Source: CAD feature listing. Evaluate the final solid. Frame: model axes, mm. A direction names the side the tool comes from. Give positions to 0.01 mm unless a question says otherwise; leave off trailing zeros. Write each loop counter-clockwise with the first axis right and the second up, starting at its lowest first coordinate (ties: lowest second). Pieces come first, ordered by that corner, then holes. Notation, with made-up numbers: (89, 47) -> (112, 47) arc R22 ccw to (112, 59) -> close; hole circle Ø7 at (58, -38). An arc over 180 degrees is marked (long way). Use one line per item in the form item = value. Start each with the question number.
(1) Cut plane B-B, the plane x = 0. Output: boundary loops of the cut face in (y, z) (3 decimals), and give its area (3 significant figures).
(2) Set-up query: faces 4 (the face through (24, 4, -15)), 5 (the face through (20.724, 3.218, -20.751)), 6 (the face through (-21, 5.5, -21)). Return all of +Z, -Z, +X, -X, +Y, -Y with unobstructed straight access to the full face (end or side cutting, diameter ignored); none if empty.
(3) Cut plane C-C, the plane x = -5. Output: boundary loops of the cut face in (y, z), and give its area (3 significant figures).
(4) Cut plane A-A, the plane y = 12. Output: boundary loops of the cut face in (x, z), and give its area (3 significant figures).
(5) Material intervals for line 1 along X through (y, z) = (14, -0.5); line 2 along Z through (x, y) = (-14, 14.5), sorted ascending. Write a range as from..to.
(6) Cut plane D-D, the plane x = 15.5. Output: boundary loops of the cut face in (y, z), and give its area (3 significant figures).
(7) Draft query along X for faces 1 (the face through (24.5, 11, 0)), 2 (the face through (-0.958, 0.493, -21.084)), 3 (the face through (24, 4, 15)). Return one class per face: pulls with the +X half, pulls with the -X half, needs draft (parallel to the pull), parting line crosses it, or undercut.
(8) First-contact query: P1, Ø0.6, axis at x = -23.5, y = 11, coming from the +Z side; P2, Ø1.5, axis at x = -17, z = -4, coming from the +Y side; P3, Ø1.5, axis at x = 13.5, z = -19.5, coming from the -Y side; P4, Ø0.5, axis at y = 4, z = -22.5, coming from the +X side. Flat tips, straight axial feed; report the tip coordinate or a pass-through.
from build123d import *

# Parameters (mm, degrees)
EXTRUDE_1_DEPTH                = 19
SKETCH_1_3_R                   = 1.75
EXTRUDE_1_2_DEPTH              = 1
HOLE_WIZARD_M2_5_1_D           = 3.1
HOLE_WIZARD_M2_5_1_DEPTH       = 10
HOLE_WIZARD_M2_5_1_CSINK_D     = 5.5
HOLE_WIZARD_M2_5_1_CSINK_ANGLE = 90
HOLE_WIZARD_M2_5_1_TIP         = 0.931333959
SKETCH_4_R                     = 2.5
SKETCH_4_R_2                   = 1.75
SKETCH_4_W                     = 27
SKETCH_4_H                     = 26.512923835
CUT_EXTRUDE_1_DEPTH            = 143
CUT_EXTRUDE_2_DEPTH            = 21
CUT_EXTRUDE_4_DEPTH            = 27
EXTRUDE_2_DEPTH                = 4.5
CUT_EXTRUDE_START              = -0.8
SKETCH_9_W                     = 7.872983346
SKETCH_9_H                     = 13
SKETCH_9_W_2                   = 6.872983346
CUT_EXTRUDE_5_DEPTH            = 0.8


with BuildPart() as part:
    # 草图1 → Extrude 1 (new body)
    with BuildSketch(Plane(origin=(0, 0, 0), x_dir=(1, 0, 0), z_dir=(0, 1, 0))):
        with BuildLine():
            Line((-24.5, 21.2), (-24.5, -21.2))
            ThreePointArc((-24.5, -21.2), (-23.533452378, -23.533452378), (-21.2, -24.5))
            Line((-21.2, -24.5), (21.2, -24.5))
            ThreePointArc((21.2, -24.5), (23.533452378, -23.533452378), (24.5, -21.2))
            Line((24.5, -21.2), (24.5, 21.2))
            ThreePointArc((24.5, 21.2), (23.533452378, 23.533452378), (21.2, 24.5))
            Line((21.2, 24.5), (-21.2, 24.5))
            ThreePointArc((-21.2, 24.5), (-23.533452378, 23.533452378), (-24.5, 21.2))
        make_face()
        with BuildLine():
            Line((-23, 21.2), (-23, -21.2))
            ThreePointArc((-23, -21.2), (-22.472792206, -22.472792206), (-21.2, -23))
            Line((-21.2, -23), (21.2, -23))
            ThreePointArc((21.2, -23), (22.472792206, -22.472792206), (23, -21.2))
            Line((23, -21.2), (23, 21.2))
            ThreePointArc((23, 21.2), (22.472792206, 22.472792206), (21.2, 23))
            Line((21.2, 23), (-21.2, 23))
            ThreePointArc((-21.2, 23), (-22.472792206, 22.472792206), (-23, 21.2))
        make_face(mode=Mode.SUBTRACT)
    extrude(amount=EXTRUDE_1_DEPTH)

    # 草图1<3> → Extrude 1 2 (add)
    with BuildSketch(Plane(origin=(0, 0, 0), x_dir=(1, 0, 0), z_dir=(0, 1, 0))):
        with BuildLine():
            Line((-21.2, -23), (21.2, -23))
            ThreePointArc((21.2, -23), (22.472792206, -22.472792206), (23, -21.2))
            Line((23, -21.2), (23, 21.2))
            ThreePointArc((23, 21.2), (22.472792206, 22.472792206), (21.2, 23))
            Line((21.2, 23), (-21.2, 23))
            ThreePointArc((-21.2, 23), (-22.472792206, 22.472792206), (-23, 21.2))
            Line((-23, 21.2), (-23, -21.2))
            ThreePointArc((-23, -21.2), (-22.472792206, -22.472792206), (-21.2, -23))
        make_face()
        with Locations(Location((-19.5, 19.5, 0), (0, 0, 270))):
            Circle(SKETCH_1_3_R, mode=Mode.SUBTRACT)
        with Locations(Location((19.5, 19.5, 0), (0, 0, 270))):
            Circle(SKETCH_1_3_R, mode=Mode.SUBTRACT)
        with Locations(Location((19.5, -19.5, 0), (0, 0, 270))):
            Circle(SKETCH_1_3_R, mode=Mode.SUBTRACT)
        with Locations(Location((-19.5, -19.5, 0), (0, 0, 270))):
            Circle(SKETCH_1_3_R, mode=Mode.SUBTRACT)
    extrude(amount=EXTRUDE_1_2_DEPTH)

    # M2.5 平头机械螺钉的锥形沉头孔1
    with Locations(Plane(origin=(-19.5, 0, 19.5), x_dir=(0, 0, -1), z_dir=(0, -1, 0))):
        with Locations((0, 0), (0, 39), (39, 39), (39, 0)):
            CounterSinkHole(HOLE_WIZARD_M2_5_1_D / 2, HOLE_WIZARD_M2_5_1_CSINK_D / 2, depth=HOLE_WIZARD_M2_5_1_DEPTH, counter_sink_angle=HOLE_WIZARD_M2_5_1_CSINK_ANGLE)
            with Locations((0, 0, -(HOLE_WIZARD_M2_5_1_DEPTH + HOLE_WIZARD_M2_5_1_TIP / 2))):  # 118° drill point
                Cone(0, HOLE_WIZARD_M2_5_1_D / 2, HOLE_WIZARD_M2_5_1_TIP, mode=Mode.SUBTRACT)

    # 草图4 → 切除-拉伸1 (cut)
    with BuildSketch(Plane.XZ):
        with Locations(Location((-11.3, -18.775, 0), (0, 0, 270))):
            Circle(SKETCH_4_R)
        with Locations(Location((0, -18.775, 0), (0, 0, 270))):
            Circle(SKETCH_4_R)
        with Locations(Location((12.3, -18.775, 0), (0, 0, 270))):
            Circle(SKETCH_4_R)
        with Locations((-19.5, -19.5)):
            Circle(SKETCH_4_R_2)
        with Locations((0, 6.876225995)):
            Rectangle(SKETCH_4_W, SKETCH_4_H)
        with BuildLine():
            Line((7.2, -13.65), (9.8, -13.65))
            ThreePointArc((9.8, -13.65), (10.65, -14.5), (9.8, -15.35))
            Line((9.8, -15.35), (7.2, -15.35))
            ThreePointArc((7.2, -15.35), (6.35, -14.5), (7.2, -13.65))
        make_face()
        with BuildLine():
            Line((-9.8, -13.65), (-7.2, -13.65))
            ThreePointArc((-7.2, -13.65), (-6.35, -14.5), (-7.2, -15.35))
            Line((-7.2, -15.35), (-9.8, -15.35))
            ThreePointArc((-9.8, -15.35), (-10.65, -14.5), (-9.8, -13.65))
        make_face()
    extrude(amount=-CUT_EXTRUDE_1_DEPTH, mode=Mode.SUBTRACT)

    # 草图5 → 切除-拉伸2 (cut)
    with BuildSketch(Plane.ZY.offset(24.5)):
        with BuildLine():
            Line((-16.186491673, 3.5), (-9.313508327, 3.5))
            ThreePointArc((-9.313508327, 3.5), (-9.265940607, 3.747991415), (-9.25, 4))
            ThreePointArc((-9.25, 4), (-9.835786438, 5.414213562), (-11.25, 6))
            Line((-11.25, 6), (-14.25, 6))
            ThreePointArc((-14.25, 6), (-15.664213562, 5.414213562), (-16.25, 4))
            ThreePointArc((-16.25, 4), (-16.234059393, 3.747991415), (-16.186491673, 3.5))
        make_face()
        with BuildLine():
            Line((-6.936491673, 3.5), (6.936491673, 3.5))
            ThreePointArc((6.936491673, 3.5), (6.58113883, 5.224744871), (5, 6))
            Line((5, 6), (-5, 6))
            ThreePointArc((-5, 6), (-6.58113883, 5.224744871), (-6.936491673, 3.5))
        make_face()
        with BuildLine():
            Line((-5, 2), (5, 2))
            ThreePointArc((5, 2), (6.224744871, 2.41886117), (6.936491673, 3.5))
            Line((6.936491673, 3.5), (-6.936491673, 3.5))
            ThreePointArc((-6.936491673, 3.5), (-6.224744871, 2.41886117), (-5, 2))
        make_face()
        with BuildLine():
            Line((8.313508327, 3.5), (16.186491673, 3.5))
            ThreePointArc((16.186491673, 3.5), (16.234059393, 3.747991415), (16.25, 4))
            ThreePointArc((16.25, 4), (15.664213562, 5.414213562), (14.25, 6))
            Line((14.25, 6), (10.25, 6))
            ThreePointArc((10.25, 6), (8.835786438, 5.414213562), (8.25, 4))
            ThreePointArc((8.25, 4), (8.265940607, 3.747991415), (8.313508327, 3.5))
        make_face()
        with BuildLine():
            Line((-16.25, 6), (-16.25, 4))
            ThreePointArc((-16.25, 4), (-15.664213562, 5.414213562), (-14.25, 6))
            Line((-14.25, 6), (-16.25, 6))
        make_face()
        with BuildLine():
            ThreePointArc((14.25, 6), (15.664213562, 5.414213562), (16.25, 4))
            Line((16.25, 4), (16.25, 6))
            Line((16.25, 6), (14.25, 6))
        make_face()
        with BuildLine():
            ThreePointArc((-11.25, 6), (-9.835786438, 5.414213562), (-9.25, 4))
            Line((-9.25, 4), (-9.25, 6))
            Line((-9.25, 6), (-11.25, 6))
        make_face()
        with BuildLine():
            Line((8.25, 6), (8.25, 4))
            ThreePointArc((8.25, 4), (8.835786438, 5.414213562), (10.25, 6))
            Line((10.25, 6), (8.25, 6))
        make_face()
    extrude(amount=-CUT_EXTRUDE_2_DEPTH, mode=Mode.SUBTRACT)

    # 草图7 → 切除-拉伸4 (cut)
    with BuildSketch(Plane(origin=(24.5, 0, 0), x_dir=(0, 0, -1), z_dir=(1, 0, 0))):
        with BuildLine():
            Line((-13, 6), (13, 6))
            ThreePointArc((13, 6), (15, 4), (13, 2))
            Line((13, 2), (-13, 2))
            ThreePointArc((-13, 2), (-15, 4), (-13, 6))
        make_face()
    extrude(amount=-CUT_EXTRUDE_4_DEPTH, mode=Mode.SUBTRACT)

    # 草图8 → 凸台-拉伸2 (add)
    with BuildSketch(Plane(origin=(0, 1, 0), x_dir=(1, 0, 0), z_dir=(0, 1, 0))):
        with BuildLine():
            Line((-23, 19.5), (-21.25, 19.5))
            ThreePointArc((-21.25, 19.5), (-20.737436867, 20.737436867), (-19.5, 21.25))
            Line((-19.5, 21.25), (-19.5, 23))
            Line((-19.5, 23), (-21.2, 23))
            ThreePointArc((-21.2, 23), (-22.472792206, 22.472792206), (-23, 21.2))
            Line((-23, 21.2), (-23, 19.5))
        make_face()
        with BuildLine():
            Line((-21.25, -19.5), (-23, -19.5))
            Line((-23, -19.5), (-23, -21.2))
            ThreePointArc((-23, -21.2), (-22.472792206, -22.472792206), (-21.2, -23))
            Line((-21.2, -23), (-19.5, -23))
            Line((-19.5, -23), (-19.5, -21.25))
            ThreePointArc((-19.5, -21.25), (-20.737436867, -20.737436867), (-21.25, -19.5))
        make_face()
        with BuildLine():
            Line((19.5, -21.25), (19.5, -23))
            Line((19.5, -23), (21.2, -23))
            ThreePointArc((21.2, -23), (22.472792206, -22.472792206), (23, -21.2))
            Line((23, -21.2), (23, -19.5))
            Line((23, -19.5), (21.25, -19.5))
            ThreePointArc((21.25, -19.5), (20.737436867, -20.737436867), (19.5, -21.25))
        make_face()
        with BuildLine():
            Line((21.2, 23), (19.5, 23))
            Line((19.5, 23), (19.5, 21.25))
            ThreePointArc((19.5, 21.25), (20.737436867, 20.737436867), (21.25, 19.5))
            Line((21.25, 19.5), (23, 19.5))
            Line((23, 19.5), (23, 21.2))
            ThreePointArc((23, 21.2), (22.472792206, 22.472792206), (21.2, 23))
        make_face()
    extrude(amount=EXTRUDE_2_DEPTH)

    # 草图9 → 切除-拉伸5 (cut)
    with BuildSketch(Plane(origin=(-23, 0, 0), x_dir=(0, 0, -1), z_dir=(1, 0, 0)).offset(CUT_EXTRUDE_START)):
        with BuildLine():
            Line((-7, 19), (-7, 4))
            ThreePointArc((-7, 4), (-6.414213562, 5.414213562), (-5, 6))
            Line((-5, 6), (5, 6))
            ThreePointArc((5, 6), (6.414213562, 5.414213562), (7, 4))
            Line((7, 4), (7, 19))
            Line((7, 19), (-7, 19))
        make_face()
        with Locations((-12.25, 12.5)):
            Rectangle(SKETCH_9_W, SKETCH_9_H)
        with Locations((12.75, 12.5)):
            Rectangle(SKETCH_9_W_2, SKETCH_9_H)
    extrude(amount=CUT_EXTRUDE_5_DEPTH, mode=Mode.SUBTRACT)


solid = part.part
Geometry says:
q1.outline = (0, -24.5) -> (19, -24.5) -> (19, -23) -> (1, -23) -> (1, -21.275) -> (0, -21.275) -> close; (0, -16.275) -> (1, -16.275) -> (1, -6.38) -> (0, -6.38) -> close; (0, 20.133) -> (1, 20.133) -> (1, 23) -> (19, 23) -> (19, 24.5) -> (0, 24.5) -> close
q1.area = 71.5 mm^2
q2.face_4 = +X
q2.face_5 = +Y, -Y
q2.face_6 = +Y
q3.outline = (0, -24.5) -> (19, -24.5) -> (19, -23) -> (1, -23) -> (1, -6.38) -> (0, -6.38) -> close; (0, 20.13) -> (1, 20.13) -> (1, 23) -> (19, 23) -> (19, 24.5) -> (0, 24.5) -> close
q3.area = 76.5 mm^2
q4.outline = (-24.5, -21.2) arc R3.3 ccw to (-21.2, -24.5) -> (21.2, -24.5) arc R3.3 ccw to (24.5, -21.2) -> (24.5, 21.2) arc R3.3 ccw to (21.2, 24.5) -> (-21.2, 24.5) arc R3.3 ccw to (-24.5, 21.2) -> close; hole (-23.8, -16.19) -> (-23, -16.19) -> (-23, -21.2) arc R1.8 ccw to (-21.2, -23) -> (21.2, -23) arc R1.8 ccw to (23, -21.2) -> (23, 21.2) arc R1.8 ccw to (21.2, 23) -> (-21.2, 23) arc R1.8 ccw to (-23, 21.2) -> (-23, 16.19) -> (-23.8, 16.19) -> (-23.8, 8.31) -> (-23, 8.31) -> (-23, 7) -> (-23.8, 7) -> (-23.8, -7) -> (-23, -7) -> (-23, -9.31) -> (-23.8, -9.31) -> close
q4.area = 255 mm^2
q5.line_1 = -24.5..-23.8, 23..24.5
q5.line_2 = -24.5..-23, 23..24.5
q6.outline = (0, -24.5) -> (19, -24.5) -> (19, -23) -> (1, -23) -> (1, 23) -> (19, 23) -> (19, 24.5) -> (0, 24.5) -> close
q6.area = 103 mm^2
q7.face_1 = pulls with the +X half
q7.face_2 = undercut
q7.face_3 = needs draft
q8.P1 = 23.82
q8.P2 = 1
q8.P3 = through
q8.P4 = 24.33
